```python
from build123d import *

# Parameters (mm, degrees)
SKETCH1_W           = 100
SKETCH1_H           = 30
BOSS_EXTRUDE1_DEPTH = 20
SKETCH2_W           = 15.2
SKETCH2_H           = 15.5
CUT_EXTRUDE1_DEPTH  = 104.07764064
SKETCH3_W           = 11
SKETCH3_H           = 2
CUT_EXTRUDE2_DEPTH  = 104.07764064
SKETCH4_W           = 1
SKETCH4_H           = 8
CUT_EXTRUDE3_DEPTH  = 104.07764064
CUT_EXTRUDE4_DEPTH  = 104.07764064
BOSS_EXTRUDE2_REACH = 104.622
SKETCH6_W           = 5
SKETCH6_H           = 17.2
FILLET1_R           = 1.5875
FILLET2_R           = 1.5875
SKETCH7_W           = 3
SKETCH7_H           = 24
CUT_EXTRUDE5_DEPTH  = 2
FILLET3_R           = 1.5875
BOSS_EXTRUDE3_DEPTH = 15.5
SKETCH9_R           = 1.905
CUT_EXTRUDE6_DEPTH  = 105.864197894
FILLET4_R           = 5
SKETCH10_R          = 2
CUT_EXTRUDE7_DEPTH  = 101.436547133


# Some blends are built 0.0001 mm under size
with BuildPart() as part:
    # Sketch1 → Boss-Extrude1 (new body)
    with BuildSketch(Plane(origin=(0, 0, 0), x_dir=(1, 0, 0), z_dir=(0, 1, 0))):
        with Locations((50, 0)):
            Rectangle(SKETCH1_W, SKETCH1_H)
    extrude(amount=BOSS_EXTRUDE1_DEPTH)

    # Sketch2 → Cut-Extrude1 (cut, through all)
    with BuildSketch(Plane.ZY):
        with Locations((0, 17.75)):
            Rectangle(SKETCH2_W, SKETCH2_H)
    extrude(amount=-CUT_EXTRUDE1_DEPTH, mode=Mode.SUBTRACT)

    # Sketch3 → Cut-Extrude2 (cut, through all)
    with BuildSketch(Plane.ZY):
        with Locations((0, 9)):
            Rectangle(SKETCH3_W, SKETCH3_H)
    extrude(amount=-CUT_EXTRUDE2_DEPTH, mode=Mode.SUBTRACT)

    # Sketch4 → Cut-Extrude3 (cut, through all)
    with BuildSketch(Plane.ZY):
        with Locations((8.1, 16)):
            Rectangle(SKETCH4_W, SKETCH4_H)
        with Locations((-8.1, 16)):
            Rectangle(SKETCH4_W, SKETCH4_H)
    extrude(amount=-CUT_EXTRUDE3_DEPTH, mode=Mode.SUBTRACT)

    # Sketch5 → Cut-Extrude4 (cut, through all)
    with BuildSketch(Plane(origin=(100, 0, 0), x_dir=(0, 0, -1), z_dir=(1, 0, 0))):
        Polygon((-12, 17.5), (12, 17.5), (12, 15.5), (15, 15.5), (15, 17.5), (15, 20), (-15, 20), (-15, 17.5), (-15, 15.5), (-12, 15.5), align=None)
    extrude(amount=-CUT_EXTRUDE4_DEPTH, mode=Mode.SUBTRACT)

    # Sketch6 → Boss-Extrude2 (add, up to next)
    with BuildSketch(Plane(origin=(0, 17.5, 0), x_dir=(1, 0, 0), z_dir=(0, 1, 0)), mode=Mode.PRIVATE) as boss_extrude2_sk1:
        with Locations((2.5, 0)):
            Rectangle(SKETCH6_W, SKETCH6_H)
    boss_extrude2_tool1 = extrude(boss_extrude2_sk1.sketch, amount=-BOSS_EXTRUDE2_REACH, mode=Mode.PRIVATE) - part.part
    add(boss_extrude2_tool1.solids().sort_by_distance((2.5, 17.5, 0))[0])

    # Fillet1
    fillet1_edges = [part.edges().sort_by_distance(p)[0] for p in [
        (5, 9, 5.5),
        (5, 14.75, 8.6),
        (5, 9, -5.5),
        (5, 14.75, -8.6),
    ]]
    fillet(fillet1_edges, radius=FILLET1_R)

    # Fillet2
    # the kernel refuses this fillet: 1.5875 mm, written as the material it adds along each edge
    with BuildSketch(Plane(origin=(5.11271188, 12, 7.6), x_dir=(1, 0, 0), z_dir=(0, -1, 0))) as fillet2_piece_1:
        with BuildLine():
            CenterArc((1.47478812, -1.5875), FILLET2_R, 90, 90)
            Line((-0.11271188, -1.5875), (-0.27146188, -1.5875))
            ThreePointArc((-0.27146188, -1.5875), (-0.27146188, -0.5875), (-0.147478812, 0.05875))
            Line((-0.147478812, 0.05875), (0, 0.15875))
            Line((0, 0.15875), (1.47478812, 0.15875))
            Line((1.47478812, 0.15875), (1.47478812, 0))
        make_face()
    extrude(amount=5.97874055)
    with BuildSketch(Plane(origin=(5.11271188, 12, -7.6), x_dir=(1, 0, 0), z_dir=(0, -1, 0))) as fillet2_piece_2:
        with BuildLine():
            CenterArc((1.47478812, 1.5875), FILLET2_R, 180, 90)
            Line((-0.11271188, 1.5875), (-0.27146188, 1.5875))
            ThreePointArc((-0.27146188, 1.5875), (-0.27146188, 0.5875), (-0.147478812, -0.05875))
            Line((-0.147478812, -0.05875), (0, -0.15875))
            Line((0, -0.15875), (1.47478812, -0.15875))
            Line((1.47478812, -0.15875), (1.47478812, 0))
        make_face()
    extrude(amount=5.97874055)

    # Sketch7 → Cut-Extrude5 (cut)
    with BuildSketch(Plane(origin=(0, 17.5, 0), x_dir=(1, 0, 0), z_dir=(0, 1, 0))):
        with Locations((1.5, 0)):
            Rectangle(SKETCH7_W, SKETCH7_H)
    extrude(amount=-CUT_EXTRUDE5_DEPTH, mode=Mode.SUBTRACT)

    # Fillet3
    fillet3_edges = [part.edges().sort_by_distance(p)[0] for p in [
        (3, 16.5, 12),
        (3, 16.5, -12),
    ]]
    fillet(fillet3_edges, radius=FILLET3_R)

    # Sketch8 → Boss-Extrude3 (add)
    with BuildSketch(Plane.XZ):
        with BuildLine():
            Line((15, 15), (15, 20))
            ThreePointArc((15, 20), (22.5, 27.5), (30, 20))
            Line((30, 20), (30, 15))
            Line((30, 15), (15, 15))
        make_face()
        with BuildLine():
            Line((70, 15), (70, 20))
            ThreePointArc((70, 20), (77.5, 27.5), (85, 20))
            Line((85, 20), (85, 15))
            Line((85, 15), (70, 15))
        make_face()
    boss_extrude3 = extrude(amount=-BOSS_EXTRUDE3_DEPTH)

    # Mirror1: Boss-Extrude3 across plane
    add(boss_extrude3.mirror(Plane.XY))

    # Sketch9 → Cut-Extrude6 (cut, through all)
    with BuildSketch(Plane(origin=(0, 15.5, 0), x_dir=(1, 0, 0), z_dir=(0, 1, 0))):
        with Locations(Location((22.5, 20, 0), (0, 0, 270))):
            Circle(SKETCH9_R)
        with Locations(Location((77.5, 20, 0), (0, 0, 270))):
            Circle(SKETCH9_R)
        with Locations(Location((77.5, -20, 0), (0, 0, 270))):
            Circle(SKETCH9_R)
        with Locations(Location((22.5, -20, 0), (0, 0, 270))):
            Circle(SKETCH9_R)
    extrude(amount=-CUT_EXTRUDE6_DEPTH, mode=Mode.SUBTRACT)

    # Fillet4
    fillet4_edges = [part.edges().sort_by_distance(p)[0] for p in [
        (15, 7.75, 15),
        (30, 7.75, 15),
        (70, 7.75, 15),
        (85, 7.75, 15),
        (85, 7.75, -15),
        (70, 7.75, -15),
        (30, 7.75, -15),
        (15, 7.75, -15),
    ]]
    fillet(fillet4_edges, radius=FILLET4_R - 0.0001)  # a hair under: the kernel refuses the full size

    # Sketch10 → Cut-Extrude7 (cut, through all)
    with BuildSketch(Plane(origin=(5, 0, 0), x_dir=(0, 0, -1), z_dir=(1, 0, 0))):
        with Locations((0, 10)):
            Circle(SKETCH10_R)
    extrude(amount=-CUT_EXTRUDE7_DEPTH, mode=Mode.SUBTRACT)


solid = part.part
```
Work out the finished part from the listing and answer in its coordinate system (mm). A direction names the side the tool comes from. Give positions to 0.01 mm unless a question says otherwise; leave off trailing zeros. Loops run counter-clockwise (first coordinate to the right, second up) from the corner with the lowest first, then second, coordinate; pieces in that order, holes last. Notation, with made-up numbers: (18, -29) -> (72, -29) arc R16 ccw to (72, -9) -> close; hole circle Ø5 at (5.25, 35.25). An arc over 180 degrees is marked (long way). Write item = value, one per line. Start each with the question number.
(1) Given pin 1 Ø0.6 at (x, y) = (44, 9) entering from -Z; pin 2 Ø1.3 at (x, z) = (40.5, -7) entering from +Y; pin 3 Ø2 at (y, z) = (8, -21.5) entering from -X, each flat-ended and moving along its own axis, determine where each tip first touches the part or whether it passes through.
(2) Find section D-D on x = 49.5. Give the vertices of the cut face in (y, z), and give its area (3 significant figures).
(3) Find section B-B on y = 5. Give the number of separate pieces and of enclosed holes in the cut face, and give its area (3 significant figures).
(4) Which of the six approach directions +Z, -Z, +X, -X, +Y, -Y give full straight-line access (tool end or side, diameter ignored) to faces 1 (the flat face through (5, 8, 15)), 2 (the flat face through (95, 8, -15)), 3 (the flat face through (5, 8, -15)), 4 (the cylindrical face through (32, 8, 16)), 5 (the flat face through (53, 12, -8))?
(5) The mould has two halves that part along Z. Classify faces 6 (the flat face through (50.2, 15.5, 12.4)), 7 (the flat face through (53, 15, -8.6)), 8 (the flat face through (50, 8, -15)), 9 (the cylindrical face through (3, 12, 0)): +Z half, -Z half, draft (parallel to the pull), parting line (faces both ways), or undercut.
(6) Find the intervals of material crossed by probe 1 along X at (y, z) = (12, -20) (3 decimals); probe 2 along X at (y, z) = (13.5, -21.5); probe 3 along Z at (x, y) = (2.6, 10), in increasing order. Write a range as from..to.
(7) Find section C-C on z = -1. Give the vertices of the cut face in (x, y).
(8) Find section A-A on x = 77.5. Give the vertices of the cut face in (y, z) (3 decimals).
From the geometry:
q1.pin_1 = -15
q1.pin_2 = 12
q1.pin_3 = 15.02
q2.outline = (0, -15) -> (15.5, -15) -> (15.5, -12) -> (17.5, -12) -> (17.5, -8.6) -> (12, -8.6) -> (12, -7.6) -> (10, -7.6) -> (10, -5.5) -> (8, -5.5) -> (8, 5.5) -> (10, 5.5) -> (10, 7.6) -> (12, 7.6) -> (12, 8.6) -> (17.5, 8.6) -> (17.5, 12) -> (15.5, 12) -> (15.5, 15) -> (0, 15) -> close
q2.area = 366 mm^2
q3.separate_pieces = 1
q3.enclosed_holes = 4
q3.area = 3,650 mm^2
q4.face_1 = +Z, -X, +Y, -Y
q4.face_2 = -Z, +X, +Y, -Y
q4.face_3 = -Z, -X, +Y, -Y
q4.face_4 = +Z, +Y, -Y
q4.face_5 = +X, +Y
q5.face_6 = draft
q5.face_7 = undercut
q5.face_8 = -Z half
q5.face_9 = undercut
q6.probe_1 = 15..20.595, 24.405..30, 70..75.595, 79.405..85
q6.probe_2 = 15.15..21.33, 23.67..29.85, 70.15..76.33, 78.67..84.85
q6.probe_3 = -15..-2, 2..15
q7.outline = (0, 0) -> (100, 0) -> (100, 8) -> (5, 8) -> (5, 8.27) -> (0, 8.27) -> close; (0, 11.73) -> (5, 11.73) -> (5, 17.5) -> (3, 17.5) -> (3, 15.5) -> (0, 15.5) -> close
q8.outline = (0, -27.5) -> (15.5, -27.5) -> (15.5, -21.905) -> (0, -21.905) -> close; (0, -18.095) -> (15.5, -18.095) -> (15.5, -12) -> (17.5, -12) -> (17.5, -8.6) -> (12, -8.6) -> (12, -7.6) -> (10, -7.6) -> (10, -5.5) -> (8, -5.5) -> (8, 5.5) -> (10, 5.5) -> (10, 7.6) -> (12, 7.6) -> (12, 8.6) -> (17.5, 8.6) -> (17.5, 12) -> (15.5, 12) -> (15.5, 18.095) -> (0, 18.095) -> close; (0, 21.905) -> (15.5, 21.905) -> (15.5, 27.5) -> (0, 27.5) -> close
